Answer from the drawing. Dimensions are ordinates in mm from the lowest x, y and z of the part. A direction names the side the tool comes from. Coordinates: 2 decimals unless noted, no trailing zeros. Write each loop counter-clockwise with the first axis right and the second up, starting at its lowest first coordinate (ties: lowest second). Pieces come first, ordered by that corner, then holes. Notation, with made-up numbers: (28.5, 18.5) -> (53.5, 18.5) arc R23 ccw to (53.5, 49.5) -> close; hole circle Ø10 at (69, 28). An arc over 180 degrees is marked (long way). Answer as a JSON object with one key per item and string values. Group by question number.
(1) Which of the six approach directions +Z, -Z, +X, -X, +Y, -Y give full straight-line access (tool end or side, diameter ignored) to the marked faces 1, 2, 3, 4 and 5?
(2) Find section B-B (z = 19.5). Give the vertices of the cut face in (x, y) (1 decimal), then the cut area to 3 significant figures.
(3) For a pull along X with two mould halves and no side action, classify the marked faces 6, 7, 8 and 9 as +X half, -X half, draft (parallel to the pull), parting line (faces both ways), or undercut.
(4) Find section A-A (y = 2.25). Give the vertices of the cut face in (x, z).
(5) Straight lines are drawn through the part: L1, parallel to Z at x = 34, y = 25.25; L2, parallel to Z at x = 21, y = 15; L3, parallel to Y at x = 37, z = 16. For each, find the intervals that lie inside material, in ascending order.
(6) Flat-ended cylindrical pins translate along their axes: P1, Ø4, axis at x = 29.5, z = 16, coming from the +Y side; P2, Ø2, axis at x = 22.5, y = 17.5, coming from the +Z side; P3, Ø14.5, axis at x = 49.5, y = 25, coming from the -Z side; P4, Ø10, axis at y = 17.5, z = 5, coming from the -X side. Find the tip coordinate at first contact, or state that the pin passes through.
(7) Find section D-D (y = 25.5). Give the vertices of the cut face in (x, z).
(8) Find section C-C (x = 11.5). Give the vertices of the cut face in (y, z).
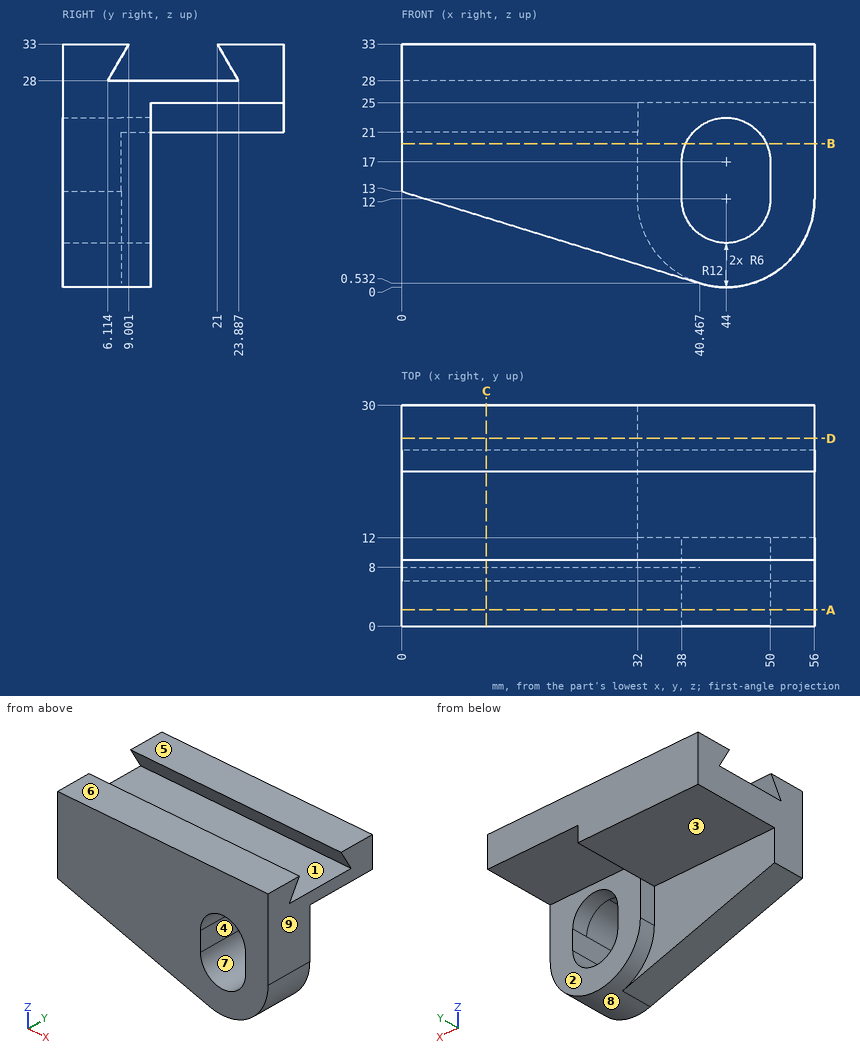
Results below:
{
 "1": {"face 1": "+X, -X", "face 2": "-Z, +X, +Y", "face 3": "-Z, -X, +Y", "face 4": "+Y, -Y", "face 5": "+Z, +X, -X, +Y, -Y"},
 "2": {"outline": "(0, 0) -> (38.5, 0) -> (38.5, 12) -> (32, 12) -> (32, 8) -> (0, 8) -> close; (49.5, 0) -> (56, 0) -> (56, 12) -> (49.5, 12) -> close", "area": "413 mm2"},
 "3": {"face 6": "draft", "face 7": "undercut", "face 8": "parting line", "face 9": "+X half"},
 "4": {"outline": "(0, 13) -> (40.47, 0.53) arc R12 ccw to (56, 12) -> (56, 33) -> (0, 33) -> close; hole (38, 12) arc R6 ccw to (50, 12) -> (50, 17) arc R6 ccw to (38, 17) -> close"},
 "5": {"L1": "z = 25 to 33", "L2": "z = 21 to 28", "L3": "y = 0 to 12"},
 "6": {"P1": "stops at y = 8", "P2": "stops at z = 28", "P3": "stops at z = 25", "P4": "passes through"},
 "7": {"outline": "(0, 21) -> (32, 21) -> (32, 25) -> (56, 25) -> (56, 33) -> (0, 33) -> close"},
 "8": {"outline": "(0, 9.46) -> (8, 9.46) -> (8, 21) -> (30, 21) -> (30, 33) -> (21, 33) -> (23.89, 28) -> (6.11, 28) -> (9, 33) -> (0, 33) -> close"}
}
